```python
from build123d import *

# Parameters (mm, degrees)
F0_R     = 3.96875
F0_R_2   = 3.175
F0_R_3   = 32.385
F0_R_4   = 19.05
F0_R_5   = 30.95625
F1_DEPTH = 9.525


with BuildPart() as f1:
    # F0 (on Front) → F1 (new body)
    with BuildSketch(Plane.XZ):
        Polygon((-76.2, 0), (0, 0), (76.2, 0), (203.2, 165.1), (203.2, 266.7), (152.4, 317.5), (0, 317.5), (-152.4, 317.5), (-203.2, 266.7), (-203.2, 165.1), align=None)
        with Locations((-30.86963, 19.93037)):
            Circle(F0_R, mode=Mode.SUBTRACT)
        with Locations((-30.86963, 81.66963)):
            Circle(F0_R, mode=Mode.SUBTRACT)
        with Locations((-101.6, 137.715625)):
            Circle(F0_R_2, mode=Mode.SUBTRACT)
        with Locations((30.86963, 19.93037)):
            Circle(F0_R, mode=Mode.SUBTRACT)
        with Locations((0, 50.8)):
            Circle(F0_R_3, mode=Mode.SUBTRACT)
        with Locations((30.86963, 81.66963)):
            Circle(F0_R, mode=Mode.SUBTRACT)
        with Locations((-179.784375, 215.9)):
            Circle(F0_R_2, mode=Mode.SUBTRACT)
        with Locations((-101.6, 215.9)):
            Circle(F0_R_4, mode=Mode.SUBTRACT)
        with Locations((-23.415625, 215.9)):
            Circle(F0_R_2, mode=Mode.SUBTRACT)
        with Locations((-101.6, 294.084375)):
            Circle(F0_R_2, mode=Mode.SUBTRACT)
        with Locations((64.690625, 173.99)):
            Circle(F0_R, mode=Mode.SUBTRACT)
        with Locations((138.509375, 173.99)):
            Circle(F0_R, mode=Mode.SUBTRACT)
        with Locations((101.6, 215.9)):
            Circle(F0_R_5, mode=Mode.SUBTRACT)
        with Locations((44.45, 250.19)):
            Circle(F0_R, mode=Mode.SUBTRACT)
        with Locations((158.75, 250.19)):
            Circle(F0_R, mode=Mode.SUBTRACT)
    extrude(amount=F1_DEPTH)


solid = f1.part
```
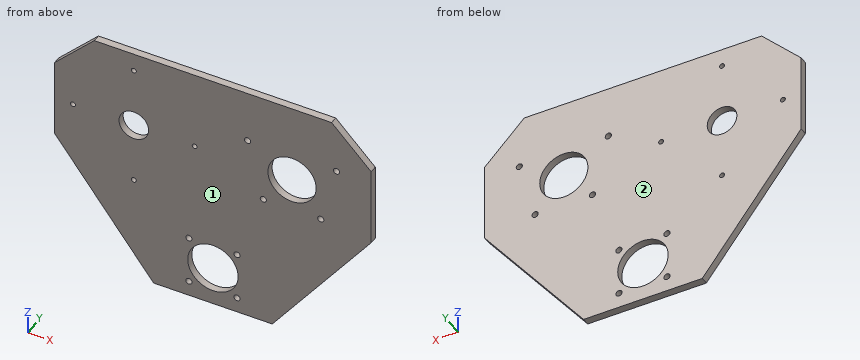
Geometry: final body of the model. Coordinates: model frame, mm. Face numbers are marked on the shaded views. Coordinates: 2 decimals unless noted, no trailing zeros. Order: outer loops, then holes, each group sorted by start corner. A loop starts at its lowest first (then second) coordinate and runs counter-clockwise, first axis right, second up. Notation, with made-up numbers: (42, -12) - (72, -12) arc R21 ccw to (72, 2) - close; hole circle Ø7 at (61, -26). An arc over 180 degrees is marked (long way). Return JSON: item names as keys, results as strings. Group by question number.
1. Cut plane A-A (x = 101.6). Output: boundary loops of the cut face in (y, z) (3 decimals).
2. Pull-direction query (Y, two-part tool) for the marked faces 1 and 2; classes: pulls with the +Y half, pulls with the -Y half, needs draft (parallel to the pull), parting line crosses it, or undercut.
3. Material intervals for line 1 along X through (y, z) = (-4, 226); line 2 along Z through (x, y) = (-101.6, -3); line 3 along X through (y, z) = (-6.5, 79), sorted ascending. Write a range as [from, to].
4. Cut plane C-C (z = 50.8). Output: boundary loops of the cut face in (x, y) (3 decimals), plus the area to 3 significant figures.
5. Cut plane B-B (y = -6). Count the separate pieces of the cut face and the enclosed holes in it, plus the area to 3 significant figures.
6. Pin query (flat end, axial travel): pin 1 (5 mm diameter, centred on x = 158.75, z = 250.19, fed in from +Y); pin 2 (3 mm diameter, centred on y = -7, z = 34, fed in from -X). Return the tip coordinate at first contact, or that it passes through.
7. Cut plane D-D (z = 130). Output: boundary loops of the cut face in (x, y) (3 decimals).
Resolved:
{
 "1": {"outline": "(-9.525, 33.02) - (0, 33.02) - (0, 184.944) - (-9.525, 184.944) - close; (-9.525, 246.856) - (0, 246.856) - (0, 317.5) - (-9.525, 317.5) - close"},
 "2": {"face 1": "pulls with the -Y half", "face 2": "pulls with the +Y half"},
 "3": {"line 1": "x = [-203.2, -117.75], [-85.45, 72.34], [130.86, 203.2]", "line 2": "z = [33.02, 134.54], [140.89, 196.85], [234.95, 290.91], [297.26, 317.5]", "line 3": "x = [-136.97, -33.81], [-27.93, -15.92], [15.92, 27.93], [33.81, 136.97]"},
 "4": {"outline": "(-115.277, -9.525) - (-32.385, -9.525) - (-32.385, 0) - (-115.277, 0) - close; (32.385, -9.525) - (115.277, -9.525) - (115.277, 0) - (32.385, 0) - close", "area": "1,580 mm²"},
 "5": {"separate pieces": "1", "enclosed holes": "15", "area": "97,500 mm²"},
 "6": {"pin 1": "passes through", "pin 2": "stops at x = -103.51"},
 "7": {"outline": "(-176.2, -9.525) - (176.2, -9.525) - (176.2, 0) - (-176.2, 0) - close"}
}
